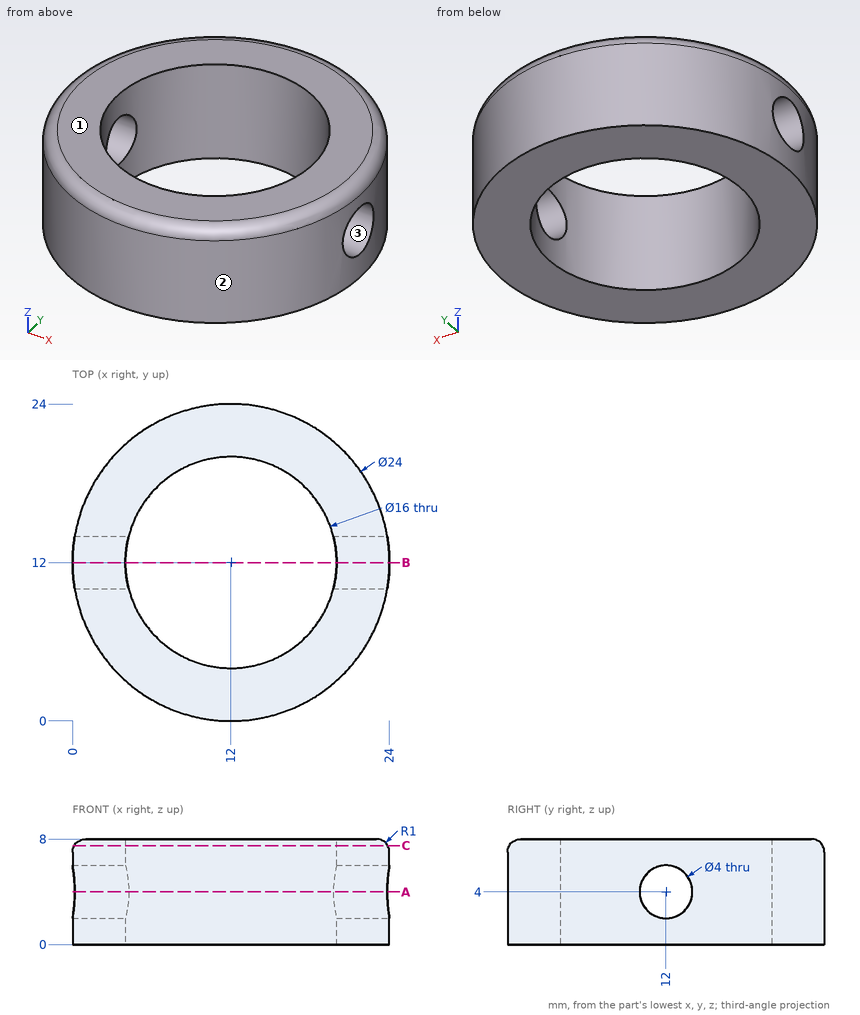
The drawing under review shows one solid part. Ordinate dimensions are in mm from its lowest x, y, z. Round coordinates to 2 decimals unless told otherwise and drop trailing zeros. Order: outer loops, then holes, each group sorted by start corner. A loop starts at its lowest first (then second) coordinate and runs counter-clockwise, first axis right, second up. Notation, with made-up numbers: (60.25, 34.5) - (66.25, 34.5) arc R7 cw to (66.25, 43.5) - close; hole circle Ø11 at (-20.75, 84.25). An arc over 180 degrees is marked (long way). Return JSON: item names as keys, results as strings.
Q1. Consider section A-A on z = 4. Write out the cut boundary in (x, y).
Computed values:
{"outline": "(0.17, 10) arc R12 ccw to (23.83, 10) - (19.75, 10) arc R8 cw to (4.25, 10) - close; (0.17, 14) - (4.25, 14) arc R8 cw to (19.75, 14) - (23.83, 14) arc R12 ccw to start"}
Q2. The part is to be moulded in two halves that separate along Y. For the marked faces 1, 2 and 3, say which applies: pulls with the +Y half, pulls with the -Y half, needs draft (parallel to the pull), parting line crosses it, or undercut.
Computed values:
{"face 1": "needs draft", "face 2": "parting line crosses it", "face 3": "undercut"}
Q3. Consider section C-C on z = 7.5. Write out the cut boundary in (x, y), plus the area to 3 significant figures.
Computed values:
{"outline": "circle Ø23.73 at (12, 12); hole circle Ø16 at (12, 12)", "area": "241 mm2"}
Q4. For pin 1 Ø1.5 at (x, z) = (4, 5.5) entering from -Y; pin 2 Ø3.5 at (y, z) = (12, 4) entering from -X; pin 3 Ø3 at (x, z) = (20, 6.5) entering from -Y; pin 4 Ø1 at (y, z) = (14.5, 1) entering from +X, all flat-tipped, find the tip position at first contact; note any pin that passes through.
Computed values:
{"pin 1": "stops at y = 2.44", "pin 2": "passes through", "pin 3": "stops at y = 1.91", "pin 4": "stops at x = 23.83"}
Q5. Consider section B-B on y = 12. Give the number of separate pieces and of enclosed holes in the cut face, plus the area to 3 significant figures.
Computed values:
{"separate pieces": "4", "enclosed holes": "0", "area": "31.6 mm2"}
Q6. Wall thickness on L1, parallel to Y at x = 12, z = 5; L2, parallel to X at y = 15, z = 2.5; L3, parallel to Y at x = 9.5, z = 5.75: over which ranges is each line inside the solid? List them lowest first. Write a range as [from, to].
Computed values:
{"L1": "y = [0, 4], [20, 24]", "L2": "x = [0.38, 4.58], [19.42, 23.62]", "L3": "y = [0.26, 4.4], [19.6, 23.74]"}
